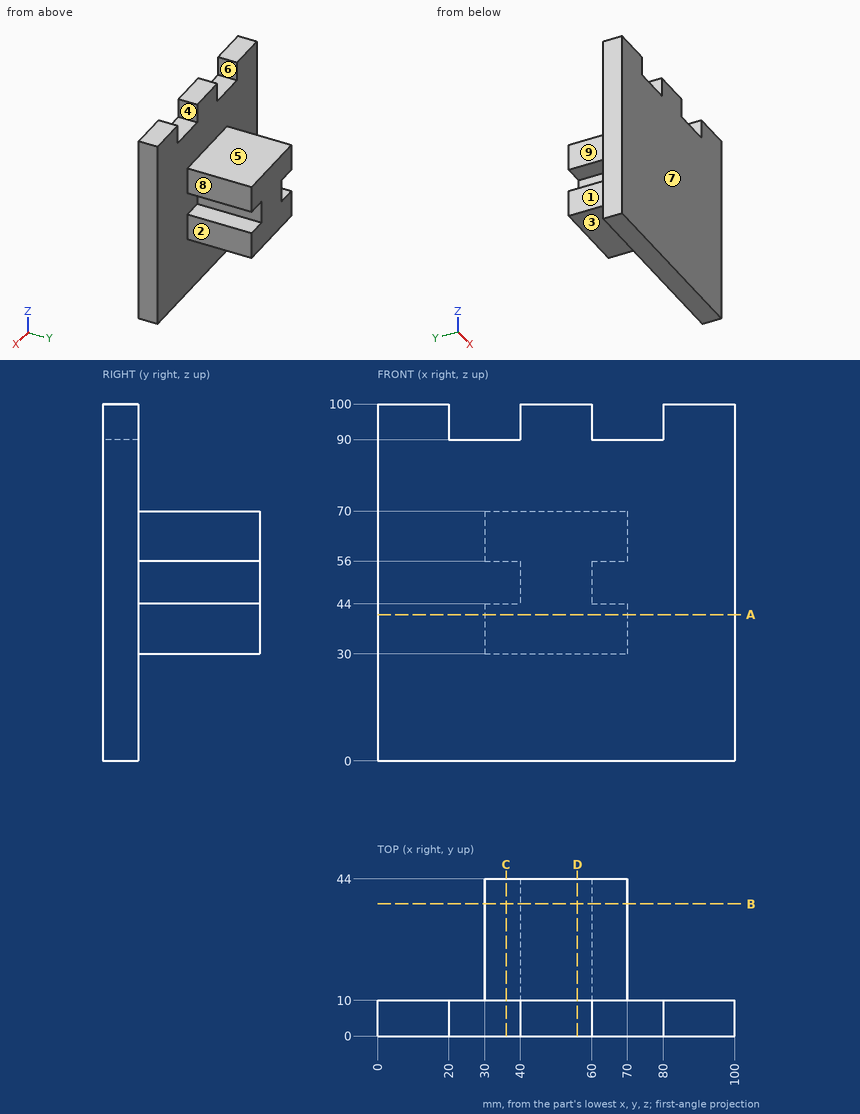
Geometry: see drawing. Coordinates: mm, zero at the bounding-box minimum. A direction names the side the tool comes from. Give positions to 0.01 mm unless a question says otherwise; leave off trailing zeros. Loops run counter-clockwise (first coordinate to the right, second up) from the corner with the lowest first, then second, coordinate; pieces in that order, holes last. Notation, with made-up numbers: M 19,-29.5 L 59,-29.5 A20 cw 59,4.5 Z; hole C 88,10 d2. An arc over 180 degrees is marked long. Use one line per item in the form item = value.
1. Section query D-D, the plane x = 56. Return the cut outline in (y, z).
Numbers:
outline = M 0,0 L 10,0 L 10,30 L 44,30 L 44,70 L 10,70 L 10,100 L 0,100 Z
2. Section query A-A, the plane z = 41. Return the cut outline in (x, y), and give its area (3 significant figures).
Numbers:
outline = M 0,0 L 100,0 L 100,10 L 70,10 L 70,44 L 30,44 L 30,10 L 0,10 Z
area = 2,360 mm²
3. Section query C-C, the plane x = 36. Return the cut outline in (y, z).
Numbers:
outline = M 0,0 L 10,0 L 10,30 L 44,30 L 44,44 L 10,44 L 10,56 L 44,56 L 44,70 L 10,70 L 10,90 L 0,90 Z
4. First-contact query: pin 1 (12 mm diameter, centred on x = 39.5, y = 23.5, fed in from +Z); pin 2 (2 mm diameter, centred on y = 27, z = 47, fed in from -X); pin 3 (4 mm diameter, centred on y = 35, z = 61.5, fed in from -X); pin 4 (11 mm diameter, centred on y = 3.5, z = 94, fed in from -X). Flat tips, straight axial feed; report the tip coordinate or a pass-through.
Numbers:
pin_1 = 70
pin_2 = 40
pin_3 = 30
pin_4 = 0
5. Pull-direction query (X, two-part tool) for the marked faces 1, 2, 3 and 4; classes: released by +X, released by -X, zero draft, split by the parting line, or undercut.
Numbers:
face_1 = released by -X
face_2 = released by +X
face_3 = zero draft
face_4 = undercut
6. Line query: L1, parallel to Z at x = 64.5, y = 18; L2, parallel to Z at x = 46.5, y = 39; L3, parallel to Y at x = 22, z = 44. Output: solid intervals per line, ascending.
Numbers:
L1 = 30 to 44, 56 to 70
L2 = 30 to 70
L3 = 0 to 10
7. Reachability of the marked faces 5, 6, 7, 8 and 9 from +Z, -Z, +X, -X, +Y, -Y: full face, straight path, thin tool, end or side. Return the list, or none.
Numbers:
face_5 = +Z, +X, -X, +Y
face_6 = +Z, +Y, -Y
face_7 = +Z, -Z, +X, -X, -Y
face_8 = +Z, -Z, +X, +Y
face_9 = +Z, -Z, -X, +Y
8. Section query B-B, the plane y = 37. Return the cut outline in (x, z), and give its area (3 significant figures).
Numbers:
outline = M 30,30 L 70,30 L 70,44 L 60,44 L 60,56 L 70,56 L 70,70 L 30,70 L 30,56 L 40,56 L 40,44 L 30,44 Z
area = 1,360 mm²
